For this review, take the finished solid that the model builds, in its own axes (mm). A direction names the side the tool comes from. Coordinates: 2 decimals unless noted, no trailing zeros. Loops run counter-clockwise (first coordinate to the right, second up) from the corner with the lowest first, then second, coordinate; pieces in that order, holes last. Notation, with made-up numbers: M -13,53.25 L 43,53.25 A34 cw 43,91.25 Z; hole C 79,42 d8. An arc over 180 degrees is marked long. Answer as a JSON object with one key per item and string values. Group by question number.
Item 1: Mouldability with a two-part tool opening along Z and no side actions: class faces 1 (the face through (-13.542, 0.098, 2.24)), 2 (the face through (-21.5, 0, 1)), 3 (the face through (-21, 0, 3)) as +Z half, -Z half, draft (parallel to the pull), parting line (faces both ways), or undercut.
Item 2: Wall thickness on L1, parallel to Y at x = 0.5, z = 1.7; L2, parallel to X at y = 9.6, z = 0.6; L3, parallel to Y at x = -18.5, z = 2.6: over which ranges is each line inside the solid? List them lowest first. Write a range as from..to.
Item 3: Add section B-B (x = -14.5). State the section outline as (y, z) points.
Item 4: Add section D-D (x = 5). State the section outline as (y, z) points.
Item 5: Add section A-A (y = 9.6). State the section outline as (x, z) points.
Item 6: Insertion check: pin 1 (1.5 mm diameter, centred on x = 11.5, y = -11.5, fed in from -Z); pin 2 (3.5 mm diameter, centred on x = -18, y = 1, fed in from +Z); pin 3 (3.5 mm diameter, centred on x = 17.72, y = -14.52, fed in from +Z). Each pin has a flat end and moves straight along its axis. Give the tip position at first contact, or say it passes through.
Item 7: Tool access review of faces 4 (the face through (-20.542, 0.098, 2.24)), 5 (the face through (21.5, 0, 1)), 6 (the face through (-4, 8, 1)), 7 (the face through (1.32, 0.1, 0.74)): name each direction out of +Z, -Z, +X, -X, +Y, -Y from which nothing blocks a thin tool from reaching the whole face with its end or side.
Item 8: Add section C-C (z = 2.4). Count the separate pieces of the cut face and the enclosed holes in it, then the cut area to 3 significant figures.
Autodesk Inventor part; units mm, degrees
ref_plane "YZ Plane" through (0, 0, 0) normal (1, 0, 0) x (0, 1, 0)
ref_plane "XZ Plane" through (0, 0, 0) normal (0, 1, 0) x (-1, 0, 0)
ref_plane "XY Plane" through (0, 0, 0) normal (0, 0, 1) x (1, 0, 0)
sketch "Sketch1" plane through (0, 0, 0) normal (0, 0, 1) x (1, 0, 0)
  circle A0 centre (17.7236, 9.6) radius 1.6
  circle A1 centre (17.7236, -14.5236) radius 1.6
  line L0 (7.5226, -3.6515) -> (7.5226, 2.8)
  line L1 (7.5226, -3.6515) -> (9.3355, -5.4645)
  arc A2 (1.9766, -12.2221) -> (9.3355, -5.4645) centre (5.8, -9) ccw
  spline S0 degree 2 poles (1.9766, -12.2221) (-3.2, -10.4641) (-8.3766, -12.2221) knots 0.21241 0.21241 0.21241 0.78759 0.78759 0.78759
  arc A3 (-15.4221, -5.1766) -> (-8.3766, -12.2221) centre (-12.2, -9) ccw
  spline S1 degree 2 poles (-15.4221, -5.1766) (-13.6641, 0) (-15.4221, 5.1766) knots 0.212408 0.212408 0.212408 0.787591 0.787591 0.787591
  arc A4 (-8.6645, 12.5355) -> (-15.4221, 5.1766) centre (-12.2, 9) ccw
  line L2 (-8.6645, 12.5355) -> (-5.3142, 9.1853)
  arc A5 (-5.3142, 9.1853) -> (-2.6505, 9.0378) centre (-3.9, 10.5995) ccw
  arc A6 (-2.6505, 9.0378) -> (-2.5046, 9) centre (-2.5046, 9.3) ccw
  line L3 (-2.5046, 9) -> (-1.9, 9)
  arc A7 (3.1749, 12.6) -> (-1.9, 9) centre (7.9405, 0.505) ccw
  line L4 (3.1749, 12.6) -> (15.5327, 12.6)
  arc A8 (15.7904, 11.8941) -> (15.5327, 12.6) centre (15.5327, 12.2) ccw
  arc A9 (15.7904, 11.8941) -> (17.7236, 6.6) centre (17.7236, 9.6) ccw
  line L5 (18.5, 6.6) -> (17.7236, 6.6)
  line L6 (18.5, 6.6) -> (18.5, 2.8)
  line L7 (7.5226, 2.8) -> (18.5, 2.8)
  line L8 (-18.5, -18.3) -> (18.5, -18.3)
  arc A10 (18.5, -18.3) -> (21.5, -15.3) centre (18.5, -15.3) ccw
  line L9 (21.5, -15.3) -> (21.5, 15.3)
  arc A11 (21.5, 15.3) -> (18.5, 18.3) centre (18.5, 15.3) ccw
  line L10 (18.5, 18.3) -> (-18.5, 18.3)
  arc A12 (-18.5, 18.3) -> (-21.5, 15.3) centre (-18.5, 15.3) ccw
  line L11 (-21.5, 15.3) -> (-21.5, -15.3)
  arc A13 (-21.5, -15.3) -> (-18.5, -18.3) centre (-18.5, -15.3) ccw
  line L12 (-21.5, 0) -> (-21.5, -8)
  line L13 (-21.5, -8) -> (-21.5, -7)
  line L14 (-21.5, -7) -> (21.5, -7)
  line L15 (-21.5, -8) -> (21.5, -8)
  line L16 (-21.5, -7) -> (14.5, -7)
  line L17 (14.5, -8) -> (14.5, 0)
  line L18 (14.5, 0) -> (-21.5, 0)
  line L19 (-21.5, -15.3) -> (-21.5, 15.3)
  line L20 (-21.5, 7) -> (21.5, 7)
  line L21 (-21.5, 8) -> (21.5, 8)
  line L22 (14.5, 8) -> (14.5, 0)
  point P0 (0, 0)
  point P1 (10.699, -8)
  point P2 (14.5, 7)
  point P3 (10.3826, -7)
  dimension "d0" = 8
  dimension "d1" = 1
  dimension "d2" = 36
extrude "Extrusion1" add sketch "Sketch1" along normal blind 3 contours L21 A9 A8 L4 A7 L3 A6 A5 L2 A4 L11 A12 L10 A11 L9 | L21 L9 L20 A9 | L21 A4 L2 A5 A6 L3 A7 L4 A8 A9 | A9 L20 L22 L21 | L20 L9 L14 L17 L22 L7 L6 L5 A9 | A9 L5 L6 L7 L22 L20 | L22 L7 L0 L18 S1 A4 L20 | L9 L15 L17 L14 | A4 S1 L18 L11 L20 | L22 L18 L0 L7 | L9 A10 L8 A13 L11 L15 A3 S0 A2 | L14 A2 L1 L0 L18 L17 | L14 A3 S1 L18 L0 L1 A2 | S1 A3 L14 L11 L18 | A2 S0 A3 L15
chamfer "Chamfer1" distance 1.5 angle 45 2 edges at (16.1236, -14.5236, 3) (16.1236, 9.6, 3)
sketch "Sketch2" plane through (-21.5, 7, 0) normal (0, 1, 0) x (1, 0, 0)
  line L0 (36, 0) -> (36, -3)
  line L1 (36, 0) -> (36, -3)
  line L2 (0, -3) -> (3, -3)
  line L3 (36, 0) -> (0, 0)
  line L4 (0, 0) -> (0, -3)
  line L5 (0, -3) -> (36, -3)
  line L6 (36, -3) -> (36, 0)
  line L7 (0, -3) -> (7.914, -3)
  line L8 (3, -3) -> (40, -3)
  line L9 (0, 0) -> (0, -3)
  line L10 (0, -1.5) -> (8, -1.5)
  line L11 (8, -1.5) -> (7.914, -3)
  line L12 (0, 0) -> (10, 0)
  line L13 (0, 0) -> (36, 0)
  line L14 (10, 0) -> (36, -1.5)
  line L15 (0, -1.5) -> (1, -1.5)
  line L16 (1, -1.5) -> (0.914, -3)
  line L17 (0, -3) -> (36, -3)
  point P0 (21.5, 0)
  point P1 (7.914, -3)
  point P2 (0, -1.5)
  point P3 (0.914, -3)
  dimension "d8" = 7.914
  dimension "d9" = 8
  dimension "d10" = 10
  dimension "d14" = 1
extrude "Extrusion2" cut sketch "Sketch2" against normal up to surface (14 mm away) contours L0 L14 L3 | L5 L2 L16 L10 L11
fillet "Fillet1" radius 0.5 4 edges at (14.5, 8, 1.5) (14.5, 7, 2.25) (14.5, -7, 2.25) (14.5, -8, 1.5)
properties part number "test_akkum_shelki"
From the geometry:
{
 "1": {"face 1": "undercut", "face 2": "draft", "face 3": "+Z half"},
 "2": {"L1": "y = -18.3..-8, -7..7, 8..18.3", "L2": "x = -21.5..16.12, 19.32..21.5", "L3": "y = -18.3..-8, 8..18.3"},
 "3": {"outline": "M -18.3,0 L -8,0 L -8,3 L -18.3,3 Z; M -7,0 L 7,0 L 7,1.5 L -7,1.5 Z; M 8,0 L 18.3,0 L 18.3,3 L 8,3 Z"},
 "4": {"outline": "M -18.3,0 L -8,0 L -8,3 L -18.3,3 Z; M -7,0.95 L 7,0.95 L 7,3 L -7,3 Z; M 8,0 L 18.3,0 L 18.3,3 L 8,3 Z"},
 "5": {"outline": "M -21.5,0 L 16.12,0 L 16.12,1.5 L 14.62,3 L -21.5,3 Z; M 19.32,0 L 21.5,0 L 21.5,3 L 20.82,3 L 19.32,1.5 Z"},
 "6": {"pin 1": "stops at z = 0", "pin 2": "stops at z = 1.5", "pin 3": "stops at z = 1.66"},
 "7": {"face 4": "+Z", "face 5": "+Z, -Z, +X, +Y, -Y", "face 6": "+Z, -Z, -X", "face 7": "-Z"},
 "8": {"separate pieces": "2", "enclosed holes": "2", "area": "1,360 mm²"}
}
